```python
from build123d import *

# Parameters (mm, degrees)
F1_DEPTH = 4


# Not quite as in the source:
# - ends of sketch curves that miss each other by under 0.0002 mm in the source are joined


with BuildPart() as f1:
    # F0 (on Top) → F1 (new body)
    with BuildSketch(Plane.XY):
        with BuildLine():
            Line((-2.4992633137, 15), (-17.5086315699, 105.0827546296))
            ThreePointArc((-17.5086315699, 105.0827546296), (0, 125.75), (17.5086315699, 105.0827546296))
            Line((17.5086315699, 105.0827546296), (2.4992633137, 15))
            Line((2.4992633137, 15), (7.4992633137, 14.9999997765))
            Line((7.4992633137, 14.9999997765), (22.5086315699, 105.0827546296))
            ThreePointArc((22.5086315699, 105.0827546296), (0, 130.6968900006), (-22.5086315699, 105.0827546296))
            Line((-22.5086315699, 105.0827546296), (-7.4992633137, 15))
            Line((-7.4992633137, 15), (-2.4992633137, 15))
        make_face()
        Polygon((2.4992633137, 14.9999997765), (-2.4992633137, 14.9999997765), (-7.4992633137, 14.9999997765), (-10.0086377934, 14.9999997765), (-10.0086377934, 9.9999997765), (9.9913622066, 9.9999997765), (9.9913622066, 14.9999997765), (7.4992633137, 14.9999997765), align=None)
    extrude(amount=F1_DEPTH)


solid = f1.part
```
Model file for the job. Use its own axes, mm. A direction names the side the tool comes from. Give positions to 0.01 mm unless a question says otherwise; leave off trailing zeros. Loops run counter-clockwise (first coordinate to the right, second up) from the corner with the lowest first, then second, coordinate; pieces in that order, holes last. Notation, with made-up numbers: (36.25, 1) - (53.25, 1) arc R16 ccw to (53.25, 18) - close; hole circle Ø6 at (88.5, 80.25). An arc over 180 degrees is marked (long way). One line per item, written item: value. Start each with the question number.
1. Slice it at B-B (x = -15.5). List the corners of the cut face in (y, z), plus the area to 3 significant figures.
2. Probe L1, parallel to X at y = 108, z = 2.35; L2, parallel to X at y = 73, z = 2.85. List the from-to ranges inside material, lowest first. Write a range as from..to.
3. Pin check, flat tips, straight feed: pin 1 (0.8 mm diameter, centred on x = -8, z = 1, fed in from +Y); pin 2 (21.5 mm diameter, centred on x = 0, y = 108, fed in from +Z); pin 3 (1.5 mm diameter, centred on y = 81, z = 2.5, fed in from -X); pin 4 (1.2 mm diameter, centred on y = 11.5, z = 2, fed in from +X). Stop position of each tip, or through.
4. Slice it at C-C (z = 1.25). List the corners of the cut face in (x, y).
5. Slice it at A-A (y = 108). List the corners of the cut face in (x, z), plus the area to 3 significant figures.
6. Which spindle directions (+Z, -Z, +X, -X, +Y, -Y) get a long thin tool onto all of the face, cutting with end or side? Do faces 5 (the flat face through (9.991, 12, 2)), 6 (the cylindrical face through (-0.431, 125.745, 1.972)), 7 (the flat face through (14.9, 59.41, 1.97)). Say none if no direction does.
7. Pull direction Y, two halves, no side cores. Call faces 1 (the flat face through (0, 10, 2)), 2 (the flat face through (9, 15, 2)), 3 (the flat face through (-10.009, 13, 2)), 4 (the flat face through (10.11, 60.67, 1.97)): pulls with the +Y half, pulls with the -Y half, needs draft (parallel to the pull), parting line crosses it, or undercut.
Solution:
1. outline: (63.02, 0) - (93.03, 0) - (93.03, 4) - (63.02, 4) - close; (116.65, 0) - (124.58, 0) - (124.58, 4) - (116.65, 4) - close
1. area: 152 mm^2
2. L1: x = -22.7..-17.75, 17.75..22.7
2. L2: x = -17.16..-12.16, 12.16..17.16
3. pin 1: stops at y = 129.39
3. pin 2: passes through
3. pin 3: stops at x = -18.62
3. pin 4: stops at x = 9.99
4. outline: (-22.51, 105.08) - (-7.5, 15) - (-10.01, 15) - (-10.01, 10) - (9.99, 10) - (9.99, 15) - (7.5, 15) - (22.51, 105.08) arc R22.7 ccw (long way) to start; hole (-17.51, 105.08) - (-2.5, 15) - (2.5, 15) - (17.51, 105.08) arc R17.75 ccw (long way) to start
5. outline: (-22.7, 0) - (-17.75, 0) - (-17.75, 4) - (-22.7, 4) - close; (17.75, 0) - (22.7, 0) - (22.7, 4) - (17.75, 4) - close
5. area: 39.6 mm^2
6. face 5: +Z, -Z, +X, -Y
6. face 6: +Z, -Z
6. face 7: +Z, -Z, +X
7. face 1: pulls with the -Y half
7. face 2: undercut
7. face 3: needs draft
7. face 4: undercut
